Build history of the part. All positions in model axes, mm. Face numbers are marked on the shaded views. A direction names the side the tool comes from. Give positions to 0.01 mm unless a question says otherwise; leave off trailing zeros. Write each loop counter-clockwise with the first axis right and the second up, starting at its lowest first coordinate (ties: lowest second). Pieces come first, ordered by that corner, then holes. Notation, with made-up numbers: (-11, 74.25) -> (-6, 74.25) arc R28 ccw to (-6, 101.25) -> close; hole circle Ø11 at (-32, -2.5). An arc over 180 degrees is marked (long way). Put each result on its own line as item: value.
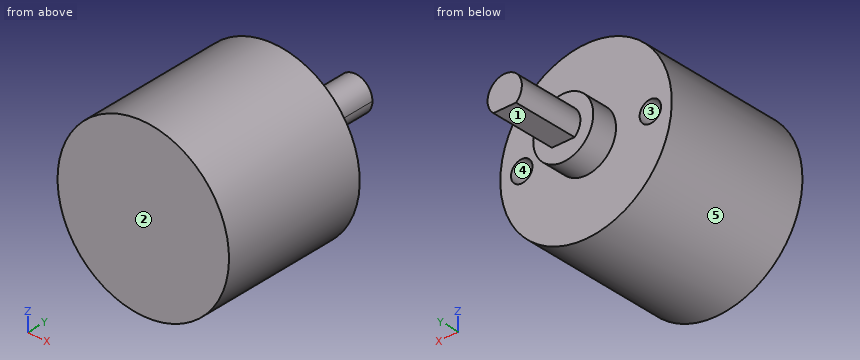
from build123d import *

# Parameters (mm, degrees)
SKETCH1_R           = 10
BOSS_EXTRUDE1_DEPTH = 17.2
SKETCH2_R           = 3.5
BOSS_EXTRUDE2_DEPTH = 3
BOSS_EXTRUDE3_DEPTH = 7.7
SKETCH4_R           = 1.25
CUT_EXTRUDE1_DEPTH  = 3.175


with BuildPart() as part:
    # Sketch1 → Boss-Extrude1 (new body)
    with BuildSketch(Plane(origin=(0, 0, 0), x_dir=(1, 0, 0), z_dir=(0, 1, 0))):
        with Locations(Location((0, 0, 0), (0, 0, 90))):
            Circle(SKETCH1_R)
    extrude(amount=BOSS_EXTRUDE1_DEPTH)

    # Sketch2 → Boss-Extrude2 (add)
    with BuildSketch(Plane(origin=(0, 17.2, 0), x_dir=(1, 0, 0), z_dir=(0, 1, 0))):
        with Locations(Location((0, 0, 0), (0, 0, 270))):
            Circle(SKETCH2_R)
    extrude(amount=BOSS_EXTRUDE2_DEPTH)

    # Sketch3 → Boss-Extrude3 (add)
    with BuildSketch(Plane(origin=(0, 20.2, 0), x_dir=(1, 0, 0), z_dir=(0, 1, 0))):
        with BuildLine():
            Line((1.322875656, 1.5), (-1.322875656, 1.5))
            ThreePointArc((-1.322875656, 1.5), (-0.822875656, -1.822875656), (2, 0))
            ThreePointArc((2, 0), (1.822875656, 0.822875656), (1.322875656, 1.5))
        make_face()
    extrude(amount=BOSS_EXTRUDE3_DEPTH)

    # Sketch4 → Cut-Extrude1 (cut)
    with BuildSketch(Plane(origin=(0, 17.2, 0), x_dir=(1, 0, 0), z_dir=(0, 1, 0))):
        with Locations(Location((-7.5, 0, 0), (0, 0, 270))):
            Circle(SKETCH4_R)
        with Locations(Location((7.5, 0, 0), (0, 0, 270))):
            Circle(SKETCH4_R)
    extrude(amount=-CUT_EXTRUDE1_DEPTH, mode=Mode.SUBTRACT)


solid = part.part
1) Pin check, flat tips, straight feed: pin 1 (1 mm diameter, centred on x = 5, y = 11.5, fed in from +Z); pin 2 (2 mm diameter, centred on x = -8, z = 0, fed in from +Y); pin 3 (3 mm diameter, centred on x = -7.5, y = 9.5, fed in from -Z). Stop position of each tip, or through.
Filled sheet:
pin 1: z = 8.93
pin 2: y = 17.2
pin 3: z = -8
2) Tool access for the marked faces 4 and 5: list every direction of +Z, -Z, +X, -X, +Y, -Y with a clear straight run to the whole face (end or side of a thin tool).
Filled sheet:
face 4: +Y
face 5: +Y, -Y
3) Wall check: L1, parallel to X at y = 15.35, z = 0; L2, parallel to Y at x = -7, z = 3; L3, parallel to Z at x = -0.25, y = 3.25. Give the ranges that are in metal, low to high.
Filled sheet:
L1: -10 to -8.75, -6.25 to 6.25, 8.75 to 10
L2: 0 to 17.2
L3: -10 to 10
4) Slice it at A-A (x = 0). Write the cut outline in (y, z), plus the area to 3 significant figures.
Filled sheet:
outline: (0, -10) -> (17.2, -10) -> (17.2, -3.5) -> (20.2, -3.5) -> (20.2, -1.5) -> (27.9, -1.5) -> (27.9, 2) -> (20.2, 2) -> (20.2, 3.5) -> (17.2, 3.5) -> (17.2, 10) -> (0, 10) -> close
area: 392 mm2
5) Slice it at D-D (x = -8.25). Write the cut outline in (y, z) (3 decimals), plus the area to 3 significant figures.
Filled sheet:
outline: (0, -5.651) -> (17.2, -5.651) -> (17.2, -1) -> (14.025, -1) -> (14.025, 1) -> (17.2, 1) -> (17.2, 5.651) -> (0, 5.651) -> close
area: 188 mm2
6) Pull direction Z, two halves, no side cores. Call the marked faces 1, 2 and 3: released by +Z, released by -Z, zero draft, split by the parting line, or undercut.
Filled sheet:
face 1: released by -Z
face 2: zero draft
face 3: undercut
7) Slice it at B-B (z = 0.5). Write the cut outline in (x, y) (1 decimal), plus the area to 3 significant figures.
Filled sheet:
outline: (-10, 0) -> (10, 0) -> (10, 17.2) -> (8.6, 17.2) -> (8.6, 14) -> (6.4, 14) -> (6.4, 17.2) -> (3.5, 17.2) -> (3.5, 20.2) -> (1.9, 20.2) -> (1.9, 27.9) -> (-1.9, 27.9) -> (-1.9, 20.2) -> (-3.5, 20.2) -> (-3.5, 17.2) -> (-6.4, 17.2) -> (-6.4, 14) -> (-8.6, 14) -> (-8.6, 17.2) -> (-10, 17.2) -> close
area: 380 mm2
8) Slice it at C-C (y = 5.25). Write the cut outline in (x, z).
Filled sheet:
outline: circle Ø20 at (0, 0)
